Source: CAD feature listing. Evaluate the final solid. Frame: model axes, mm. Round coordinates to 2 decimals unless told otherwise and drop trailing zeros. Order: outer loops, then holes, each group sorted by start corner. A loop starts at its lowest first (then second) coordinate and runs counter-clockwise, first axis right, second up. Notation, with made-up numbers: (73, -34) -> (121, -34) arc R14 ccw to (121, -20) -> close; hole circle Ø10 at (58.5, 35.5). An arc over 180 degrees is marked (long way). Use a Markdown table: item, result. Add a question column.
```python
from build123d import *

# Parameters (mm, degrees)
SKETCH1_W            = 40
SKETCH1_H            = 40
BOSS_EXTRUDE1_DEPTH  = 4.7625
M5_CLEARANCE_HOLE1_D = 5.3


with BuildPart() as part:
    # Sketch1 → Boss-Extrude1 (new body)
    with BuildSketch(Plane.XY):
        with Locations((20, 20)):
            Rectangle(SKETCH1_W, SKETCH1_H)
        with Locations((20, 60)):
            Rectangle(SKETCH1_W, SKETCH1_H)
        with Locations((60, 60)):
            Rectangle(SKETCH1_W, SKETCH1_H)
        Polygon((40, 40), (40, 0), (80, 40), align=None)
    extrude(amount=BOSS_EXTRUDE1_DEPTH)

    # M5 Clearance Hole1 (through all)
    with Locations(Plane.XY.offset(4.7625)):
        with Locations((10, 70), (30, 70), (50, 70), (70, 70), (30, 50), (50, 50), (70, 50), (30, 30), (50, 30), (30, 10), (10, 50), (10, 30), (10, 10)):
            Hole(M5_CLEARANCE_HOLE1_D / 2)


solid = part.part
```
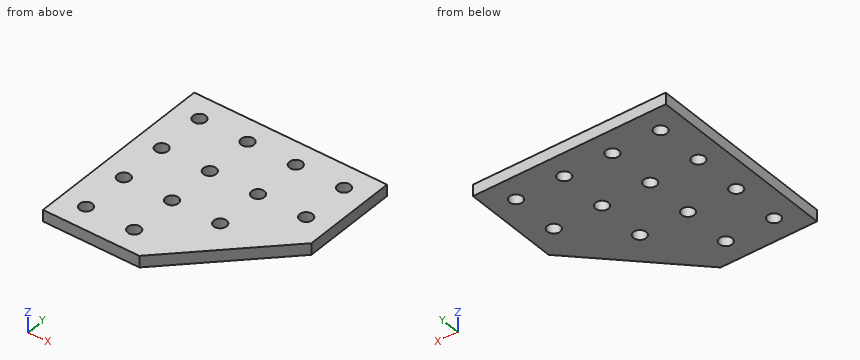
1) First-contact query: pin 1 Ø4 at (x, y) = (10, 70) entering from +Z. Flat tip, straight axial feed; report the tip coordinate or a pass-through.
2) Line query: probe 1 along Y at (x, z) = (10, 2.9); probe 2 along X at (y, z) = (68, 0.25); probe 3 along X at (y, z) = (68.5, 3.4). Output: solid intervals per line, ascending. Write a range as from..to.
3) Section A-A on y = 30. Output: boundary loops of the cut face in (x, z), then the cut area to 3 significant figures.
4) Section B-B on x = 30. Output: boundary loops of the cut face in (y, z).
5) Section C-C on z = 3.4. Count the separate pieces of the cut face and the enclosed holes in it, then the cut area to 3 significant figures.
6) Section D-D on y = 10. Output: boundary loops of the cut face in (x, z), then the cut area to 3 significant figures.
Conclusion:
| question | item | result |
|---|---|---|
| 1 | pin 1 | passes through |
| 2 | probe 1 | y = 0..7.35, 12.65..27.35, 32.65..47.35, 52.65..67.35, 72.65..80 |
| 2 | probe 2 | x = 0..8.26, 11.74..28.26, 31.74..48.26, 51.74..68.26, 71.74..80 |
| 2 | probe 3 | x = 0..7.82, 12.18..27.82, 32.18..47.82, 52.18..67.82, 72.18..80 |
| 3 | outline | (0, 0) -> (7.35, 0) -> (7.35, 4.76) -> (0, 4.76) -> close; (12.65, 0) -> (27.35, 0) -> (27.35, 4.76) -> (12.65, 4.76) -> close; (32.65, 0) -> (47.35, 0) -> (47.35, 4.76) -> (32.65, 4.76) -> close; (52.65, 0) -> (70, 0) -> (70, 4.76) -> (52.65, 4.76) -> close |
| 3 | area | 258 mm^2 |
| 4 | outline | (0, 0) -> (7.35, 0) -> (7.35, 4.76) -> (0, 4.76) -> close; (12.65, 0) -> (27.35, 0) -> (27.35, 4.76) -> (12.65, 4.76) -> close; (32.65, 0) -> (47.35, 0) -> (47.35, 4.76) -> (32.65, 4.76) -> close; (52.65, 0) -> (67.35, 0) -> (67.35, 4.76) -> (52.65, 4.76) -> close; (72.65, 0) -> (80, 0) -> (80, 4.76) -> (72.65, 4.76) -> close |
| 5 | separate pieces | 1 |
| 5 | enclosed holes | 13 |
| 5 | area | 5,310 mm^2 |
| 6 | outline | (0, 0) -> (7.35, 0) -> (7.35, 4.76) -> (0, 4.76) -> close; (12.65, 0) -> (27.35, 0) -> (27.35, 4.76) -> (12.65, 4.76) -> close; (32.65, 0) -> (50, 0) -> (50, 4.76) -> (32.65, 4.76) -> close |
| 6 | area | 188 mm^2 |
